from build123d import *

# Parameters (mm, degrees)
PAD008_DEPTH    = 3
PAD009_DEPTH    = 1.5
POCKET_DEPTH    = 5
FILLET_R        = 2
FILLET001_R     = 2
SKETCH023_R     = 2
POCKET001_DEPTH = 4.501
FILLET002_R     = 0.5


with BuildPart() as part:
    # Sketch020 → Pad008 (new body)
    with BuildSketch(Plane.XY):
        Polygon((0, 37.8364245462), (-32.7673048454, -18.9182122731), (32.7673048454, -18.9182122731), align=None)
    extrude(amount=-PAD008_DEPTH)

    # Sketch021 → Pad009 (join)
    with BuildSketch(Plane.XY):
        Polygon((0, 35.8364245464), (-31.035254038, -17.9182122732), (31.035254038, -17.9182122732), align=None)
    extrude(amount=PAD009_DEPTH)

    # Sketch022 → Pocket (cut)
    with BuildSketch(Plane.XY):
        Polygon((0, 25.8364245462), (-22.375, -12.9182122731), (22.375, -12.9182122731), align=None)
        Polygon((0, 21.8364245462), (-18.9108983849, -10.9182122731), (18.9108983849, -10.9182122731), align=None, mode=Mode.SUBTRACT)
    extrude(amount=POCKET_DEPTH, mode=Mode.SUBTRACT)

    # Fillet
    fillet_edges = [part.edges().sort_by_distance(p)[0] for p in [
        (-32.767305, -18.918212, -1.5),
        (32.767305, -18.918212, -1.5),
        (0, 37.836425, -1.5),
        (31.035254, -17.918212, 0.75),
        (-31.035254, -17.918212, 0.75),
        (0, 35.836425, 0.75),
    ]]
    fillet(fillet_edges, radius=FILLET_R)

    # Fillet001
    fillet001_edges = [part.edges().sort_by_distance(p)[0] for p in [
        (0, 21.836425, 0.75),
        (18.910898, -10.918212, 0.75),
        (-18.910898, -10.918212, 0.75),
    ]]
    fillet(fillet001_edges, radius=FILLET001_R)

    # Sketch023 (on Face11 of Fillet001) → Pocket001 (cut, through all)
    with BuildSketch(Plane.XY.offset(1.5)):
        with Locations((0, 19.8364245462)):
            Circle(SKETCH023_R)
    extrude(amount=-POCKET001_DEPTH, mode=Mode.SUBTRACT)

    # Fillet002
    fillet002_edges = [part.edges().sort_by_distance(p)[0] for p in [
        (16.383652, 9.459106, -3),
    ]]
    fillet(fillet002_edges, radius=FILLET002_R)


solid = part.part
Design review of the part built by this model. Coordinates are the model's own, in mm. A direction names the side the tool comes from. Round coordinates to 2 decimals unless told otherwise and drop trailing zeros. Loops run counter-clockwise (first coordinate to the right, second up) from the corner with the lowest first, then second, coordinate; pieces in that order, holes last. Notation, with made-up numbers: (24.25, -3.5) - (57.25, -3.5) arc R26 cw to (57.25, 13.5) - close; hole circle Ø6 at (89.5, 79.25). An arc over 180 degrees is marked (long way). One line per item, written item: value. Start each with the question number.
1) Insertion check: pin 1 Ø1.2 at (x, z) = (-13.5, 1) entering from -Y; pin 2 Ø0.8 at (x, z) = (5, 1) entering from +Y; pin 3 Ø1 at (y, z) = (20, -2) entering from -X. Each pin has a flat end and moves straight along its axis. Give the tip position at first contact, or say it passes through.
2) For faces 1 (the flat face through (9.564, 5.272, 0.74)), 2 (the flat face through (15.711, 8.625, 0.74)), 3 (the flat face through (-15.325, 9.293, 0.74)), list the 3-axis set-ups (+Z, -Z, +X, -X, +Y, -Y) from which the entire face can be reached by the end or side of a thin tool; tool diameter is ignored.
3) Draft analysis for pull direction X (two halves, no side actions). For faces 4 (the cylindrical face through (-29.32, -16.89, 0.76)), 5 (the cylindrical face through (-17.193, -9.893, 0.76)), 6 (the cylindrical face through (29.29, -16.94, 0.76)), state which applies: +X half, -X half, draft (parallel to the pull), parting line (faces both ways), or undercut.
4) To check wall thickness, follow L1, parallel to X at y = 18, z = 1.1; L2, parallel to Y at x = 0, z = -0.05; L3, parallel to X at y = 3, z = 1.3. State the ranges of each line that lie inside material, in increasing order. Write a range as from..to.
5) Consider section A-A on z = -1.15. Give the boundary of the cut face in (x, y), then the cut area to 3 significant figures.
Reported:
1. pin 1: stops at y = -17.92
1. pin 2: stops at y = 27.87
1. pin 3: stops at x = -10.59
2. face 1: +Z
2. face 2: +Z, +X, +Y
2. face 3: +Z, -X, +Y
3. face 4: -X half
3. face 5: undercut
3. face 6: +X half
4. L1: x = -10.3..-4.52, -2.21..-0.79, 0.79..2.21, 4.52..10.3
4. L2: y = -18.92..17.84, 21.84..35.84
4. L3: x = -18.96..-13.18, -10.88..10.88, 13.18..18.96
5. outline: (-31.04, -15.92) arc R2 ccw to (-29.3, -18.92) - (29.3, -18.92) arc R2 ccw to (31.04, -15.92) - (1.73, 34.84) arc R2 ccw to (-1.73, 34.84) - close; hole circle Ø4 at (0, 19.84)
5. area: 1,840 mm^2
